Build history of the part. All positions in model axes, mm. A direction names the side the tool comes from. Round coordinates to 2 decimals unless told otherwise and drop trailing zeros. Loops run counter-clockwise (first coordinate to the right, second up) from the corner with the lowest first, then second, coordinate; pieces in that order, holes last.
from build123d import *

# Parameters (mm, degrees)
SKETCH1_W           = 55
SKETCH1_H           = 32
BOSS_EXTRUDE1_DEPTH = 50
SKETCH2_W           = 45
SKETCH2_H           = 32
CUT_EXTRUDE1_DEPTH  = 45
SKETCH3_R           = 1.75
CUT_EXTRUDE2_DEPTH  = 51
SKETCH4_R           = 1.75
CUT_EXTRUDE3_DEPTH  = 56
SKETCH5_W           = 1.1
SKETCH5_H           = 35
CUT_EXTRUDE4_DEPTH  = 1.2


with BuildPart() as part:
    # Sketch1 → Boss-Extrude1 (new body)
    with BuildSketch(Plane(origin=(0, 0, 0), x_dir=(1, 0, 0), z_dir=(0, 1, 0))):
        with Locations((27.5, 16)):
            Rectangle(SKETCH1_W, SKETCH1_H)
    extrude(amount=BOSS_EXTRUDE1_DEPTH)

    # Sketch2 → Cut-Extrude1 (cut)
    with BuildSketch(Plane.XZ):
        with Locations((27.5, -16)):
            Rectangle(SKETCH2_W, SKETCH2_H)
    extrude(amount=-CUT_EXTRUDE1_DEPTH, mode=Mode.SUBTRACT)

    # Sketch3 → Cut-Extrude2 (cut, through all)
    with BuildSketch(Plane(origin=(0, 50, 0), x_dir=(1, 0, 0), z_dir=(0, 1, 0))):
        with Locations((43.5, 26)):
            Circle(SKETCH3_R)
        with Locations((43.5, 6)):
            Circle(SKETCH3_R)
        with Locations((11.5, 26)):
            Circle(SKETCH3_R)
        with Locations((11.5, 6)):
            Circle(SKETCH3_R)
    extrude(amount=-CUT_EXTRUDE2_DEPTH, mode=Mode.SUBTRACT)

    # Sketch4 → Cut-Extrude3 (cut, through all)
    with BuildSketch(Plane(origin=(55, 0, 0), x_dir=(0, 0, -1), z_dir=(1, 0, 0))):
        with Locations((6, 5)):
            Circle(SKETCH4_R)
        with Locations((26, 5)):
            Circle(SKETCH4_R)
    extrude(amount=-CUT_EXTRUDE3_DEPTH, mode=Mode.SUBTRACT)

    # Sketch5 → Cut-Extrude4 (cut)
    with BuildSketch(Plane.ZY.offset(-50)):
        with Locations((-29.45, 27.5)):
            Rectangle(SKETCH5_W, SKETCH5_H)
        with Locations((-31.45, 27.5)):
            Rectangle(SKETCH5_W, SKETCH5_H)
        with Locations((-27.45, 27.5)):
            Rectangle(SKETCH5_W, SKETCH5_H)
        with Locations((-25.45, 27.5)):
            Rectangle(SKETCH5_W, SKETCH5_H)
        with Locations((-23.45, 27.5)):
            Rectangle(SKETCH5_W, SKETCH5_H)
        with Locations((-21.45, 27.5)):
            Rectangle(SKETCH5_W, SKETCH5_H)
        with Locations((-19.45, 27.5)):
            Rectangle(SKETCH5_W, SKETCH5_H)
        with Locations((-17.45, 27.5)):
            Rectangle(SKETCH5_W, SKETCH5_H)
        with Locations((-15.45, 27.5)):
            Rectangle(SKETCH5_W, SKETCH5_H)
        with Locations((-13.45, 27.5)):
            Rectangle(SKETCH5_W, SKETCH5_H)
        with Locations((-11.45, 27.5)):
            Rectangle(SKETCH5_W, SKETCH5_H)
        with Locations((-9.45, 27.5)):
            Rectangle(SKETCH5_W, SKETCH5_H)
        with Locations((-7.45, 27.5)):
            Rectangle(SKETCH5_W, SKETCH5_H)
        with Locations((-5.45, 27.5)):
            Rectangle(SKETCH5_W, SKETCH5_H)
        with Locations((-3.45, 27.5)):
            Rectangle(SKETCH5_W, SKETCH5_H)
        with Locations((-1.45, 27.5)):
            Rectangle(SKETCH5_W, SKETCH5_H)
        with Locations((0.55, 27.5)):
            Rectangle(SKETCH5_W, SKETCH5_H)
    extrude(amount=-CUT_EXTRUDE4_DEPTH, mode=Mode.SUBTRACT)


solid = part.part
(1) Which spindle directions (+Z, -Z, +X, -X, +Y, -Y) get a long thin tool onto all of the face, cutting with end or side? Do faces 1 (the face through (5, 22, -16)), 2 (the face through (2, 0, -16)). Say none if no direction does.
Responses:
face 1: +Z, -Z, -Y
face 2: +Z, -Z, +X, -X, -Y
(2) Slice it at B-B on y = 5. List the corners of the cut face in (x, z).
Responses:
outline: (0, -32) - (5, -32) - (5, -27.75) - (0, -27.75) - close; (0, -24.25) - (5, -24.25) - (5, -7.75) - (0, -7.75) - close; (0, -4.25) - (5, -4.25) - (5, 0) - (0, 0) - close; (50, -32) - (55, -32) - (55, -27.75) - (50, -27.75) - close; (50, -24.25) - (55, -24.25) - (55, -7.75) - (50, -7.75) - close; (50, -4.25) - (55, -4.25) - (55, 0) - (50, 0) - close
(3) Pin check, flat tips, straight feed: P1, Ø2, axis at x = 43.5, z = -26, coming from the +Y side (1 decimal); P2, Ø3, axis at x = 19.5, z = -6, coming from the -Y side; P3, Ø1, axis at x = 50.5, y = 25.5, coming from the -Z side. Stop position of each tip, or through.
Responses:
P1: passes through
P2: stops at y = 45
P3: stops at z = -30.9
(4) Pull direction Y, two halves, no side cores. Call faces 3 (the face through (52.54, 3.29, -5.62)), 4 (the face through (12.31, 47.54, -4.45)), 5 (the face through (52, 0, -16)), 6 (the face through (52.54, 3.94, -24.61)): +Y half, -Y half, draft (parallel to the pull), parting line (faces both ways), or undercut.
Responses:
face 3: undercut
face 4: draft
face 5: -Y half
face 6: undercut
(5) Slice it at A-A on x = 43.5. List the corners of the cut face in (y, z).
Responses:
outline: (45, -32) - (50, -32) - (50, -27.75) - (45, -27.75) - close; (45, -24.25) - (50, -24.25) - (50, -7.75) - (45, -7.75) - close; (45, -4.25) - (50, -4.25) - (50, 0) - (45, 0) - close
(6) Slice it at C-C on x = 38. List the corners of the cut face in (y, z), plus the area to 3 significant figures.
Responses:
outline: (45, -32) - (50, -32) - (50, 0) - (45, 0) - close
area: 160 mm2
(7) Probe line 1 (X direction, y = 46.55, z = -26); line 2 (Z direction, x = 11.5, y = 48.75); line 3 (Y direction, x = 53.35, z = -6). List the from-to ranges inside material, lowest first.
Responses:
line 1: x = 0 to 9.75, 13.25 to 41.75, 45.25 to 55
line 2: z = -32 to -27.75, -24.25 to -7.75, -4.25 to 0
line 3: y = 0 to 3.25, 6.75 to 50
